Verification items for this drawing (mm, ordinates from the low corner). Round coordinates to 2 decimals unless told otherwise and drop trailing zeros. Order: outer loops, then holes, each group sorted by start corner. A loop starts at its lowest first (then second) coordinate and runs counter-clockwise, first axis right, second up. Notation, with made-up numbers: (-7, 2) -> (50, 2) arc R13 ccw to (50, 22) -> close; hole circle Ø7 at (76.5, 85). An arc over 180 degrees is marked (long way). Return JSON: item names as keys, results as strings. Group by question number.
Item 1: Sectioned sample at D-D on x = 50.5. Record the cut outline in (y, z) (3 decimals), plus the area to 4 significant figures.
Item 2: Sectioned sample at A-A on z = 62. Record the cut outline in (x, y) (3 decimals), plus the area to 3 significant figures.
Item 3: Sectioned sample at C-C on y = 1.15. Record the cut outline in (x, z) (3 decimals), plus the area to 3 significant figures.
Item 4: Depth check by flat-ended pin: pin 1 Ø1 at (x, y) = (34.5, 2.5) entering from -Z. Enter the tip coordinate at first touch or a pass-through.
Item 5: Scan lines: probe 1 along X at (y, z) = (1, 70.5); probe 2 along X at (y, z) = (2.05, 47.5) (3 decimals); probe 3 along Z at (x, y) = (160, 2.35) (3 decimals). Record each from-to range of solid material in increasing order. Write a range as from..to.
Item 6: Sectioned sample at B-B on x = 82.5. Record the cut outline in (y, z) (3 decimals), plus the area to 3 significant figures.
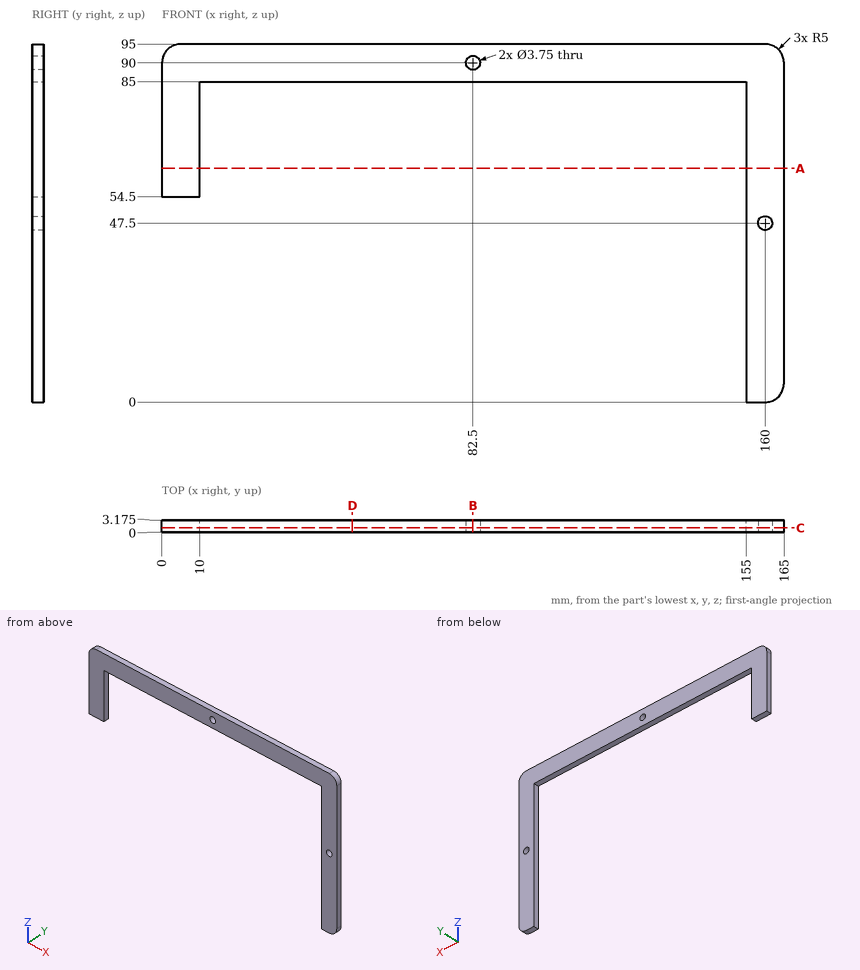
Recorded:
{
 "1": {"outline": "(0, 85) -> (3.175, 85) -> (3.175, 95) -> (0, 95) -> close", "area": "31.75 mm²"},
 "2": {"outline": "(0, 0) -> (10, 0) -> (10, 3.175) -> (0, 3.175) -> close; (155, 0) -> (165, 0) -> (165, 3.175) -> (155, 3.175) -> close", "area": "63.5 mm²"},
 "3": {"outline": "(0, 54.5) -> (10, 54.5) -> (10, 85) -> (155, 85) -> (155, 0) -> (160, 0) arc R5 ccw to (165, 5) -> (165, 90) arc R5 ccw to (160, 95) -> (5, 95) arc R5 ccw to (0, 90) -> close; hole circle Ø3.75 at (82.5, 90); hole circle Ø3.75 at (160, 47.5)", "area": "2,770 mm²"},
 "4": {"pin 1": "z = 85"},
 "5": {"probe 1": "0..10, 155..165", "probe 2": "155..158.125, 161.875..165", "probe 3": "0..45.625, 49.375..95"},
 "6": {"outline": "(0, 85) -> (3.175, 85) -> (3.175, 88.125) -> (0, 88.125) -> close; (0, 91.875) -> (3.175, 91.875) -> (3.175, 95) -> (0, 95) -> close", "area": "19.8 mm²"}
}
